from build123d import *

# Parameters (mm, degrees)
SKETCH1_W           = 52
SKETCH1_H           = 40
SKETCH1_W_2         = 48
SKETCH1_H_2         = 36
BOSS_EXTRUDE1_DEPTH = 40
SKETCH2_W           = 40
SKETCH2_H           = 2
BOSS_EXTRUDE2_DEPTH = 80
SKETCH3_R           = 4
BOSS_EXTRUDE3_DEPTH = 150


with BuildPart() as part:
    # Sketch1 → Boss-Extrude1 (new body)
    with BuildSketch(Plane(origin=(0, 0, 0), x_dir=(1, 0, 0), z_dir=(0, 1, 0))):
        with Locations((26, -20)):
            Rectangle(SKETCH1_W, SKETCH1_H)
        with Locations((26, -20)):
            Rectangle(SKETCH1_W_2, SKETCH1_H_2, mode=Mode.SUBTRACT)
    extrude(amount=BOSS_EXTRUDE1_DEPTH)

    # Sketch2 → Boss-Extrude2 (add)
    with BuildSketch(Plane(origin=(52, 0, 0), x_dir=(0, 0, -1), z_dir=(1, 0, 0))):
        with Locations((-20, 39)):
            Rectangle(SKETCH2_W, SKETCH2_H)
    extrude(amount=BOSS_EXTRUDE2_DEPTH)

    # Sketch3 → Boss-Extrude3 (add)
    with BuildSketch(Plane(origin=(52, 0, 0), x_dir=(0, 0, -1), z_dir=(1, 0, 0))):
        with Locations(Location((-20, 15, 0), (0, 0, 180))):
            Circle(SKETCH3_R)
    extrude(amount=BOSS_EXTRUDE3_DEPTH)


solid = part.part
The listing builds one solid part. Answer for the finished solid, in the listing's coordinates (mm). A direction names the side the tool comes from. Round coordinates to 2 decimals unless told otherwise and drop trailing zeros. Loops run counter-clockwise (first coordinate to the right, second up) from the corner with the lowest first, then second, coordinate; pieces in that order, holes last. Notation, with made-up numbers: M 48.5,69 L 100.5,69 A15 ccw 100.5,78 Z; hole C 82,39.25 d6. An arc over 180 degrees is marked long. Return JSON: item names as keys, results as strings.
Q1. Find the intervals of material crossed by line 1 along Z through (x, y) = (33.5, 5.5); line 2 along X through (y, z) = (17, 34); line 3 along X through (y, z) = (16.5, 20.5), in increasing order. Write a range as from..to.
Results list:
{"line 1": "z = 0..2, 38..40", "line 2": "x = 0..2, 50..52", "line 3": "x = 0..2, 50..202"}
Q2. Find section C-C, the plane y = 15. Determine the outline of the cut face in (x, z).
Results list:
{"outline": "M 0,0 L 52,0 L 52,16 L 202,16 L 202,24 L 52,24 L 52,40 L 0,40 Z; hole M 2,2 L 50,2 L 50,38 L 2,38 Z"}
Q3. Each of these flat-tipped pins is pushed along its axis until it touches: pin 1 Ø19 at (y, z) = (27, 26.5) entering from +X; pin 2 Ø8 at (x, z) = (66.5, 33) entering from -Y; pin 3 Ø0.6 at (y, z) = (39, 22) entering from +X. Where does it stop, or does it pass through?
Results list:
{"pin 1": "stops at x = 52", "pin 2": "stops at y = 38", "pin 3": "stops at x = 132"}
Q4. The mould has two halves that part along Y. Classify faces 3 (the face through (24, 0, 39)), 4 (the face through (125.95, 11.034, 19.479)), 5 (the face through (80, 40, 20)), 6 (the face through (202, 15, 20)): released by +Y, released by -Y, zero draft, split by the parting line, or undercut.
Results list:
{"face 3": "released by -Y", "face 4": "undercut", "face 5": "released by +Y", "face 6": "zero draft"}
Q5. Find section D-D, the plane z = 9.5. Determine the outline of the cut face in (x, y).
Results list:
{"outline": "M 0,0 L 2,0 L 2,40 L 0,40 Z; M 50,0 L 52,0 L 52,38 L 132,38 L 132,40 L 50,40 Z"}
Q6. Find section A-A, the plane z = 20. Determine the outline of the cut face in (x, y), plus the area to 3 significant figures.
Results list:
{"outline": "M 0,0 L 2,0 L 2,40 L 0,40 Z; M 50,0 L 52,0 L 52,11 L 202,11 L 202,19 L 52,19 L 52,38 L 132,38 L 132,40 L 50,40 Z", "area": "1,520 mm2"}
Q7. Which of the six approach directions +Z, -Z, +X, -X, +Y, -Y give full straight-line access (tool end or side, diameter ignored) to faces 1 (the face through (21, 20, 40)), 2 (the face through (26, 20, 2))?
Results list:
{"face 1": "+Z, +X, -X, +Y, -Y", "face 2": "+Y, -Y"}
Q8. Find section B-B, the plane x = 43.5. Determine the outline of the cut face in (y, z).
Results list:
{"outline": "M 0,0 L 40,0 L 40,2 L 0,2 Z; M 0,38 L 40,38 L 40,40 L 0,40 Z"}
